```python
from build123d import *

# Parameters (mm, degrees)
ESQUISSE1_R             = 9.45
BOSS_EXTRU_1_DEPTH      = 25
CONG_1_R                = 0.25
ESQUISSE2_R             = 4
ENL_V_MAT_EXTRU_1_DEPTH = 17.5
ESQUISSE3_R             = 3
ENL_V_MAT_EXTRU_2_DEPTH = 17.5
ESQUISSE4_R             = 1.5
ENL_V_MAT_EXTRU_3_DEPTH = 10
ESQUISSE5_R             = 1.5
ENL_V_MAT_EXTRU_4_DEPTH = 10
ESQUISSE7_W             = 0.372914415
ESQUISSE7_H             = 1.339729566


with BuildPart() as part:
    # Esquisse1 → Boss.-Extru.1 (new body)
    with BuildSketch(Plane.XY):
        Circle(ESQUISSE1_R)
    extrude(amount=BOSS_EXTRU_1_DEPTH)

    # Congé1
    cong_1_edges = [part.edges().sort_by_distance(p)[0] for p in [
        (-9.45, 0, 0),
        (-9.45, 0, 25),
    ]]
    fillet(cong_1_edges, radius=CONG_1_R)

    # Esquisse2 → Enlèv. mat.-Extru.1 (cut)
    with BuildSketch(Plane.XY.offset(25)):
        Circle(ESQUISSE2_R)
    extrude(amount=-ENL_V_MAT_EXTRU_1_DEPTH, mode=Mode.SUBTRACT)

    # Esquisse3 → Enlèv. mat.-Extru.2 (cut)
    with BuildSketch(Plane(origin=(0, 0, 0), x_dir=(-1, 0, 0), z_dir=(0, 0, -1))):
        Circle(ESQUISSE3_R)
    extrude(amount=-ENL_V_MAT_EXTRU_2_DEPTH, mode=Mode.SUBTRACT)

    # Esquisse4 → Enlèv. mat.-Extru.3 (cut)
    with BuildSketch(Plane(origin=(9.45, 0, 0), x_dir=(0, 0, -1), z_dir=(1, 0, 0))):
        with Locations((-4.589130857, 0.014370537)):
            Circle(ESQUISSE4_R)
        with Locations((-20.520433185, 0.068499333)):
            Circle(ESQUISSE4_R)
    extrude(amount=-ENL_V_MAT_EXTRU_3_DEPTH, mode=Mode.SUBTRACT)

    # Esquisse5 → Enlèv. mat.-Extru.4 (cut)
    with BuildSketch(Plane(origin=(0, 9.45, 0), x_dir=(1, 0, 0), z_dir=(0, 1, 0))):
        with Locations((-0.124304805, -20.496942457)):
            Circle(ESQUISSE5_R)
        with Locations((-0.124304805, -4.503057543)):
            Circle(ESQUISSE5_R)
    extrude(amount=-ENL_V_MAT_EXTRU_4_DEPTH, mode=Mode.SUBTRACT)

    # Esquisse7 → Enlèvement de matière-Révolution1 (revolve, cut)
    with BuildSketch(Plane(origin=(0, 0, 0), x_dir=(0, 0, -1), z_dir=(1, 0, 0))):
        with Locations((-12.937755344, 9.16402646)):
            Rectangle(ESQUISSE7_W, ESQUISSE7_H)
        with Locations((-14.937755344, 9.16402646)):
            Rectangle(ESQUISSE7_W, ESQUISSE7_H)
        with Locations((-10.937755344, 9.16402646)):
            Rectangle(ESQUISSE7_W, ESQUISSE7_H)
    revolve(axis=Axis((0, 0, 25), (0, 0, -1)), mode=Mode.SUBTRACT)


solid = part.part
```
Geometry: final body of the model. Coordinates: model frame, mm. A direction names the side the tool comes from. Coordinates: 2 decimals unless noted, no trailing zeros. Order: outer loops, then holes, each group sorted by start corner. A loop starts at its lowest first (then second) coordinate and runs counter-clockwise, first axis right, second up. Notation, with made-up numbers: (56.25, 48) -> (94.25, 48) arc R21 ccw to (94.25, 68) -> close; hole circle Ø5 at (33.5, 8). An arc over 180 degrees is marked (long way). Write item = value, one per line.
(1) Cut plane A-A on z = 23.5. Return loops of the section in (x, y).
Solved:
outline = circle Ø18.9 at (0, 0); hole circle Ø8 at (0, 0)
(2) Access query for faces 1 (the flat face through (4, 8, 15.124)), 2 (the cylindrical face through (1.306, 6.035, 4.052)), 3 (the cylindrical face through (-0.867, -3.905, 16.373)), 4 (the cylindrical face through (-1.384, -2.662, 3.698)), 5 (the cylindrical face through (6.068, 0.08, 6.088)). Directions: +Z, -Z, +X, -X, +Y, -Y. A direction counts if a zero-diameter tool reaches every point of the face in a straight line with its end or side. Return the directions, or none.
Solved:
face_1 = none
face_2 = +Y
face_3 = +Z
face_4 = +Z, -Z
face_5 = +X
(3) Pin query (flat end, axial travel): pin 1 Ø1 at (x, z) = (-7, 18) entering from -Y; pin 2 Ø2.5 at (x, y) = (-1.5, 1) entering from +Z; pin 3 Ø1.5 at (y, z) = (-7, 11) entering from -X; pin 4 Ø6 at (y, z) = (0.5, 10) entering from -X. Return the tip coordinate at first contact, or that it passes through.
Solved:
pin_1 = -6.86
pin_2 = 7.5
pin_3 = -7.08
pin_4 = -9.45
(4) Line query: line 1 (Z direction, x = -7.5, y = 5.5); line 2 (Z direction, x = -3.5, y = 0.25); line 3 (Z direction, x = 6, y = 0.75). Output: solid intervals per line, ascending.
Solved:
line_1 = 0.02 to 10.75, 11.12 to 12.75, 13.12 to 14.75, 15.12 to 24.98
line_2 = 0 to 7.5
line_3 = 0 to 3.28, 5.9 to 19.18, 21.86 to 25
(5) Pull-direction query (Y, two-part tool) for faces 6 (the cylindrical face through (9.014, 2.839, 11.926)), 7 (the flat face through (4, 8, 13.124)), 8 (the flat face through (1, 3, 7.5)); classes: pulls with the +Y half, pulls with the -Y half, needs draft (parallel to the pull), parting line crosses it, or undercut.
Solved:
face_6 = parting line crosses it
face_7 = needs draft
face_8 = undercut
(6) Cut plane B-B on x = 0. Count the separate pieces of the cut face and the enclosed holes in it, plus the area to 3 significant figures.
Solved:
separate_pieces = 4
enclosed_holes = 0
area = 250 mm²
